```python
from build123d import *

# Parameters (mm, degrees)
SKETCH1_W           = 60
SKETCH1_H           = 55
BOSS_EXTRUDE1_DEPTH = 11.25
SKETCH2_R           = 2.25
BOSS_EXTRUDE2_DEPTH = 6
CHAMFER1_SIZE       = 10
FILLET1_R           = 10
FILLET2_R           = 5
SKETCH3_R           = 2.5
BOSS_EXTRUDE3_DEPTH = 30


with BuildPart() as part:
    # Sketch1 → Boss-Extrude1 (new, symmetric)
    with BuildSketch(Plane(origin=(0, 0, 0), x_dir=(1, 0, 0), z_dir=(0, 1, 0))):
        Rectangle(SKETCH1_W, SKETCH1_H)
    extrude(amount=BOSS_EXTRUDE1_DEPTH, both=True)

    # Sketch2 → Boss-Extrude2 (add)
    with BuildSketch(Plane.XZ.offset(11.25)):
        with BuildLine():
            Line((-14, -27.5), (-6.641845526, -38.459359596))
            ThreePointArc((-6.641845526, -38.459359596), (0, -42), (6.641845526, -38.459359596))
            Line((6.641845526, -38.459359596), (14, -27.5))
            Line((14, -27.5), (-14, -27.5))
        make_face()
        with Locations(Location((0, -34, 0), (0, 0, 270))):
            Circle(SKETCH2_R, mode=Mode.SUBTRACT)
    boss_extrude2 = extrude(amount=-BOSS_EXTRUDE2_DEPTH)

    # Mirror1: Boss-Extrude2 across plane
    add(boss_extrude2.mirror(Plane.XY))

    # Chamfer1
    chamfer1_edges = [part.edges().sort_by_distance(p)[0] for p in [
        (-30, 0, -27.5),
        (30, 0, -27.5),
        (30, 0, 27.5),
        (-30, 0, 27.5),
    ]]
    chamfer(chamfer1_edges, length=CHAMFER1_SIZE)

    # Fillet1
    fillet1_edges = [part.edges().sort_by_distance(p)[0] for p in [
        (20, 0, 27.5),
        (-20, 0, 27.5),
        (-30, 0, -17.5),
        (-30, 0, 17.5),
        (30, 0, -17.5),
        (30, 0, 17.5),
        (-20, 0, -27.5),
        (20, 0, -27.5),
    ]]
    fillet(fillet1_edges, radius=FILLET1_R)

    # Fillet2
    # the kernel refuses this fillet: 5 mm, written as the material it adds along each edge
    with BuildSketch(Plane(origin=(14, -11.25, -27.5), x_dir=(0.9999804368407044, 0, 0.006255072811241643), z_dir=(0, 1, 0)), Plane(origin=(-14, -11.25, 27.5), x_dir=(-0.9999804368407044, 0, -0.006255072811243166), z_dir=(0, 1, 0))) as fillet2_piece_1:
        with BuildLine():
            CenterArc((2.6493765, 4.994091646), FILLET2_R, 214.235948787, 52.978387625)
            Line((-1.484262233, 2.181080656), (-1.897626106, 1.899779557))
            Line((-1.897626106, 1.899779557), (-0.413363873, -0.281301099))
            Line((-0.413363873, -0.281301099), (0.003127536, -0.499990218))
            ThreePointArc((0.003127536, -0.499990218), (1.860955567, -0.488369141), (2.382077328, -0.499409165))
            Line((2.382077328, -0.499409165), (2.406377253, 0))
        make_face()
    extrude(amount=6)
    with BuildSketch(Plane(origin=(-14, -11.25, -27.5), x_dir=(-0.9999804368407044, 0, 0.00625507281124311), z_dir=(0, 1, 0)), Plane(origin=(14, -11.25, 27.5), x_dir=(0.9999804368407044, 0, -0.006255072811241634), z_dir=(0, 1, 0))) as fillet2_piece_2:
        with BuildLine():
            CenterArc((2.6493765, -4.994091646), FILLET2_R, 92.785663588, 52.978387625)
            Line((-1.484262233, -2.181080656), (-1.897626106, -1.899779557))
            Line((-1.897626106, -1.899779557), (-0.413363873, 0.281301099))
            Line((-0.413363873, 0.281301099), (0.003127536, 0.499990218))
            ThreePointArc((0.003127536, 0.499990218), (1.860955567, 0.488369141), (2.382077328, 0.499409165))
            Line((2.382077328, 0.499409165), (2.406377253, 0))
        make_face()
    extrude(amount=6)

    # Sketch3 → Boss-Extrude3 (add)
    with BuildSketch(Plane.ZY.offset(30)):
        with Locations(Location((0, -5.25, 0), (0, 0, 180))):
            Circle(SKETCH3_R)
    extrude(amount=BOSS_EXTRUDE3_DEPTH)


solid = part.part
```
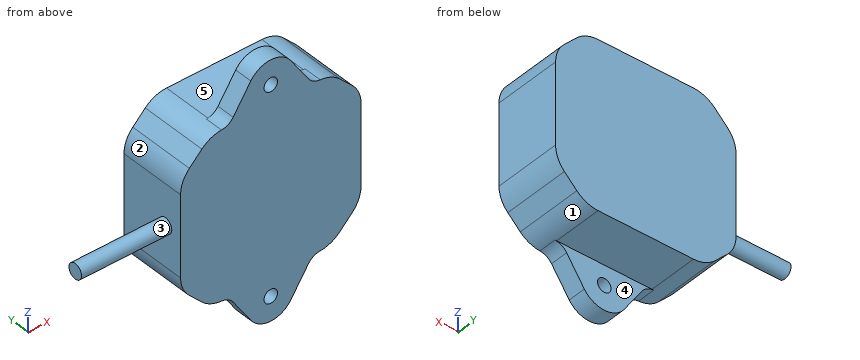
Check sheet for the modelled part. Datum: model origin and axes. Units: mm. Face numbers are marked on the shaded views. A direction names the side the tool comes from. Coordinates: 2 decimals unless noted, no trailing zeros. Write each loop counter-clockwise with the first axis right and the second up, starting at its lowest first coordinate (ties: lowest second). Pieces come first, ordered by that corner, then holes. Notation, with made-up numbers: M 72.25,-27.5 L 107.25,-27.5 A30 cw 107.25,0.5 Z; hole C 58,40 d5. An arc over 180 degrees is marked long. Use one line per item in the form item = value.
Item 1: Sectioned sample at A-A, the plane y = -9.5. Record the cut outline in (x, z).
Answer below:
outline = M -30,-13.36 A10 ccw -27.07,-20.43 L -22.93,-24.57 A10 ccw -16.41,-27.48 A5 cw -12.53,-29.69 L -6.64,-38.46 A8 ccw 6.64,-38.46 L 12.53,-29.69 A5 cw 16.41,-27.48 A10 ccw 22.93,-24.57 L 27.07,-20.43 A10 ccw 30,-13.36 L 30,13.36 A10 ccw 27.07,20.43 L 22.93,24.57 A10 ccw 16.41,27.48 A5 cw 12.53,29.69 L 6.64,38.46 A8 ccw -6.64,38.46 L -12.53,29.69 A5 cw -16.41,27.48 A10 ccw -22.93,24.57 L -27.07,20.43 A10 ccw -30,13.36 Z; hole C 0,-34 d4.5; hole C 0,34 d4.5
Item 2: Material ranges on L1, parallel to Z at x = -15, y = 5; L2, parallel to X at y = -7.6, z = 34; L3, parallel to X at y = 8.25, z = 11, recorded low to high. Write a range as from..to.
Answer below:
L1 = -27.5..27.5
L2 = -9.64..-2.25, 2.25..9.64
L3 = -30..30
Item 3: Set-up check for the marked faces 1, 2, 3, 4 and 5: record each of +Z, -Z, +X, -X, +Y, -Y from which the full face is reachable in a straight line by a thin tool's end or side.
Answer below:
face_1 = -Z, +X, +Y, -Y
face_2 = +Z, -X, +Y, -Y
face_3 = -X
face_4 = -Z, +X, -X, +Y
face_5 = +Z, +X, -X, +Y
Item 4: Sectioned sample at B-B, the plane x = 0. Record the cut outline in (y, z).
Answer below:
outline = M -11.25,-42 L -5.25,-42 L -5.25,-36.25 L -11.25,-36.25 Z; M -11.25,-31.75 L -5.25,-31.75 L -5.25,-27.5 L 11.25,-27.5 L 11.25,27.5 L -5.25,27.5 L -5.25,31.75 L -11.25,31.75 Z; M -11.25,36.25 L -5.25,36.25 L -5.25,42 L -11.25,42 Z
Item 5: Sectioned sample at C-C, the plane z = -34. Record the cut outline in (x, y), and give its area (3 significant figures).
Answer below:
outline = M -9.64,-11.25 L -2.25,-11.25 L -2.25,-5.25 L -9.64,-5.25 Z; M 2.25,-11.25 L 9.64,-11.25 L 9.64,-5.25 L 2.25,-5.25 Z
area = 88.6 mm^2
Item 6: Sectioned sample at D-D, the plane y = 9.25. Record the cut outline in (x, z).
Answer below:
outline = M -30,-13.36 A10 ccw -27.07,-20.43 L -22.93,-24.57 A10 ccw -15.86,-27.5 L 15.86,-27.5 A10 ccw 22.93,-24.57 L 27.07,-20.43 A10 ccw 30,-13.36 L 30,13.36 A10 ccw 27.07,20.43 L 22.93,24.57 A10 ccw 15.86,27.5 L -15.86,27.5 A10 ccw -22.93,24.57 L -27.07,20.43 A10 ccw -30,13.36 Z
Item 7: Gauge pin test, flat ends, axial feed: pin 1 Ø10 at (y, z) = (3.5, -1) entering from -X; pin 2 Ø5 at (x, y) = (-0.5, 2) entering from +Z; pin 3 Ø1.5 at (x, y) = (-44.5, -2.5) entering from +Z. Record the tip position at first contact, or that the pin passes through.
Answer below:
pin_1 = -30
pin_2 = 27.5
pin_3 = 1.5
